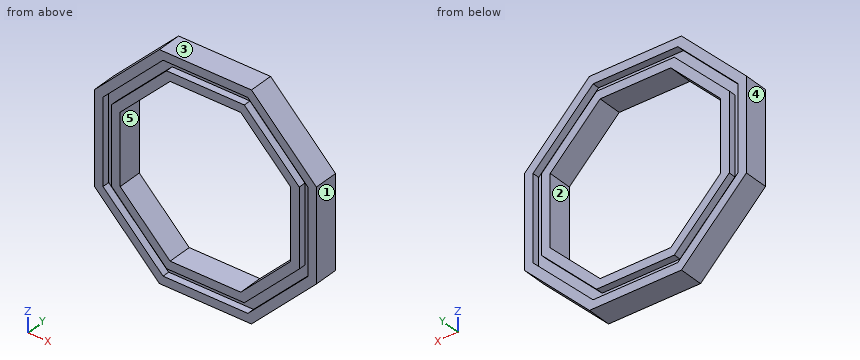
from build123d import *

# Parameters (mm, degrees)
EXTRUDE_1_DEPTH     = 1.7
CUT_EXTRUDE_3_DEPTH = 1
CUT_EXTRUDE_4_DEPTH = 2.7


with BuildPart() as part:
    # 스케치1 → 보스-돌출1 (new body)
    with BuildSketch(Plane(origin=(0, 0, 0), x_dir=(1, 0, 0), z_dir=(0, 1, 0))):
        Polygon((-15.520132754, -6.428649477), (-6.428649477, -15.520132754), (6.428649477, -15.520132754), (15.520132754, -6.428649477), (15.520132754, 6.428649477), (6.428649477, 15.520132754), (-6.428649477, 15.520132754), (-15.520132754, 6.428649477), align=None)
        Polygon((-5.931593202, -14.320132754), (5.931593202, -14.320132754), (14.320132754, -5.931593202), (14.320132754, 5.931593202), (5.931593202, 14.320132754), (-5.931593202, 14.320132754), (-14.320132754, 5.931593202), (-14.320132754, -5.931593202), align=None, mode=Mode.SUBTRACT)
        Polygon((-14.320132754, -5.931593202), (-5.931593202, -14.320132754), (5.931593202, -14.320132754), (14.320132754, -5.931593202), (14.320132754, 5.931593202), (5.931593202, 14.320132754), (-5.931593202, 14.320132754), (-14.320132754, 5.931593202), align=None)
        Polygon((-5.434536927, -13.120132754), (5.434536927, -13.120132754), (13.120132754, -5.434536927), (13.120132754, 5.434536927), (5.434536927, 13.120132754), (-5.434536927, 13.120132754), (-13.120132754, 5.434536927), (-13.120132754, -5.434536927), align=None, mode=Mode.SUBTRACT)
        Polygon((-13.120132754, -5.434536927), (-5.434536927, -13.120132754), (5.434536927, -13.120132754), (13.120132754, -5.434536927), (13.120132754, 5.434536927), (5.434536927, 13.120132754), (-5.434536927, 13.120132754), (-13.120132754, 5.434536927), align=None)
    extrude_1 = extrude(amount=EXTRUDE_1_DEPTH)

    # 스케치2 → 컷-돌출3 (cut)
    with BuildSketch(Plane(origin=(0, 1.7, 0), x_dir=(1, 0, 0), z_dir=(0, 1, 0))):
        Polygon((-14.320132754, -5.931593202), (-5.931593202, -14.320132754), (5.931593202, -14.320132754), (14.320132754, -5.931593202), (14.320132754, 5.931593202), (5.931593202, 14.320132754), (-5.931593202, 14.320132754), (-14.320132754, 5.931593202), align=None)
        Polygon((-13.120132754, -5.434536927), (-5.434536927, -13.120132754), (5.434536927, -13.120132754), (13.120132754, -5.434536927), (13.120132754, 5.434536927), (5.434536927, 13.120132754), (-5.434536927, 13.120132754), (-13.120132754, 5.434536927), align=None, mode=Mode.SUBTRACT)
    cut_extrude_3 = extrude(amount=-CUT_EXTRUDE_3_DEPTH, mode=Mode.SUBTRACT)

    # 스케치3 → 컷-돌출4 (cut, through all)
    with BuildSketch(Plane(origin=(0, 1.7, 0), x_dir=(1, 0, 0), z_dir=(0, 1, 0))):
        Polygon((-4.937480652, 11.920132754), (-11.920132754, 4.937480652), (-11.920132754, -4.937480652), (-4.937480652, -11.920132754), (4.937480652, -11.920132754), (11.920132754, -4.937480652), (11.920132754, 4.937480652), (4.937480652, 11.920132754), align=None)
    cut_extrude_4 = extrude(amount=-CUT_EXTRUDE_4_DEPTH, mode=Mode.SUBTRACT)

    # 대칭 복사1: 보스-돌출1, 컷-돌출3, 컷-돌출4 across plane
    add(extrude_1.mirror(Plane.ZX))
    add(cut_extrude_3.mirror(Plane.ZX), mode=Mode.SUBTRACT)
    add(cut_extrude_4.mirror(Plane.ZX), mode=Mode.SUBTRACT)


solid = part.part
Build history of the part. All positions in model axes, mm. Face numbers are marked on the shaded views. A direction names the side the tool comes from. Round coordinates to 2 decimals unless told otherwise and drop trailing zeros. Write each loop counter-clockwise with the first axis right and the second up, starting at its lowest first coordinate (ties: lowest second). Pieces come first, ordered by that corner, then holes. Notation, with made-up numbers: (84, 52) -> (127, 52) arc R12 cw to (127, 65) -> close; hole circle Ø1 at (-31, 53). An arc over 180 degrees is marked (long way). Use one line per item in the form item = value.
Q1. Band-saw the part on D-D, the plane x = 12.5. Write the cut outline in (y, z), then the cut area to 3 significant figures.
Conclusion:
outline = (-1.7, -9.45) -> (1.7, -9.45) -> (1.7, -7.75) -> (0.7, -7.75) -> (0.7, -6.05) -> (1.7, -6.05) -> (1.7, 6.05) -> (0.7, 6.05) -> (0.7, 7.75) -> (1.7, 7.75) -> (1.7, 9.45) -> (-1.7, 9.45) -> (-1.7, 7.75) -> (-0.7, 7.75) -> (-0.7, 6.05) -> (-1.7, 6.05) -> (-1.7, -6.05) -> (-0.7, -6.05) -> (-0.7, -7.75) -> (-1.7, -7.75) -> close
area = 57.5 mm²
Q2. Drill centre lines: L1, parallel to Z at x = 4, y = 1.4; L2, parallel to Z at x = 13, y = 0.85. Where is each one in solid material? Low to high.
Conclusion:
L1 = -15.52 to -14.32, -13.12 to -11.92, 11.92 to 13.12, 14.32 to 15.52
L2 = -8.95 to -7.25, -5.55 to 5.55, 7.25 to 8.95
Q3. Drop flat-ended pins along their axis: P1, Ø2, axis at y = 0, z = 9, coming from the -X side; P2, Ø1, axis at x = 8.5, y = 0, coming from the -Z side. Give the stop position or say it passes through.
Conclusion:
P1 = -13.95
P2 = -13.95
Q4. Two-plate mould, pull along X, no slides. Class the marked faces 1, 2 and 3: released by +X, released by -X, zero draft, split by the parting line, or undercut.
Conclusion:
face_1 = released by +X
face_2 = undercut
face_3 = zero draft
Q5. Band-saw the part on C-C, the plane x = 8.5. Write the cut outline in (y, z), then the cut area to 3 significant figures.
Conclusion:
outline = (-1.7, -13.45) -> (1.7, -13.45) -> (1.7, -11.75) -> (0.7, -11.75) -> (0.7, -10.05) -> (1.7, -10.05) -> (1.7, -8.36) -> (-1.7, -8.36) -> (-1.7, -10.05) -> (-0.7, -10.05) -> (-0.7, -11.75) -> (-1.7, -11.75) -> close; (-1.7, 8.36) -> (1.7, 8.36) -> (1.7, 10.05) -> (0.7, 10.05) -> (0.7, 11.75) -> (1.7, 11.75) -> (1.7, 13.45) -> (-1.7, 13.45) -> (-1.7, 11.75) -> (-0.7, 11.75) -> (-0.7, 10.05) -> (-1.7, 10.05) -> close
area = 27.8 mm²
Q6. Tool access for the marked faces 4 and 5: list every direction of +Z, -Z, +X, -X, +Y, -Y with a clear straight run to the whole face (end or side of a thin tool).
Conclusion:
face_4 = +Z, -Z, -X, +Y, -Y
face_5 = +Y, -Y
Q7. Band-saw the part on A-A, the plane y = -1.15. State how many separate pieces and enclosed holes the cut face has, then the cut area to 3 significant figures.
Conclusion:
separate_pieces = 2
enclosed_holes = 2
area = 218 mm²
Q8. Band-saw the part on B-B, the plane z = 2. Write the cut outline in (x, y), then the cut area to 3 significant figures.
Conclusion:
outline = (-15.52, -1.7) -> (-14.32, -1.7) -> (-14.32, -0.7) -> (-13.12, -0.7) -> (-13.12, -1.7) -> (-11.92, -1.7) -> (-11.92, 1.7) -> (-13.12, 1.7) -> (-13.12, 0.7) -> (-14.32, 0.7) -> (-14.32, 1.7) -> (-15.52, 1.7) -> close; (11.92, -1.7) -> (13.12, -1.7) -> (13.12, -0.7) -> (14.32, -0.7) -> (14.32, -1.7) -> (15.52, -1.7) -> (15.52, 1.7) -> (14.32, 1.7) -> (14.32, 0.7) -> (13.12, 0.7) -> (13.12, 1.7) -> (11.92, 1.7) -> close
area = 19.7 mm²
